Verification items for the finished model (mm, model axes). Round coordinates to 2 decimals unless told otherwise and drop trailing zeros. Order: outer loops, then holes, each group sorted by start corner. A loop starts at its lowest first (then second) coordinate and runs counter-clockwise, first axis right, second up. Notation, with made-up numbers: M -12,59 L 10,59 A27 ccw 10,96 Z; hole C 80,15 d2. An arc over 180 degrees is marked long. Use one line per item in the form item = value. Start each with the question number.
Item 1: Cross-section at A-A on z = -2. Enter the section's corners in (x, y).
Item 2: Thickness scan on probe 1 along Z at (x, y) = (249.5, -5); probe 2 along Y at (x, z) = (0, -29.35); probe 3 along Y at (x, z) = (-298.5, -6). Record the ranges inside material, lowest first. Write a range as [from, to].
Item 3: Cross-section at B-B on x = 680. Enter the section's corners in (y, z).
Item 4: Cross-section at C-C on x = -46. Enter the section's corners in (y, z).
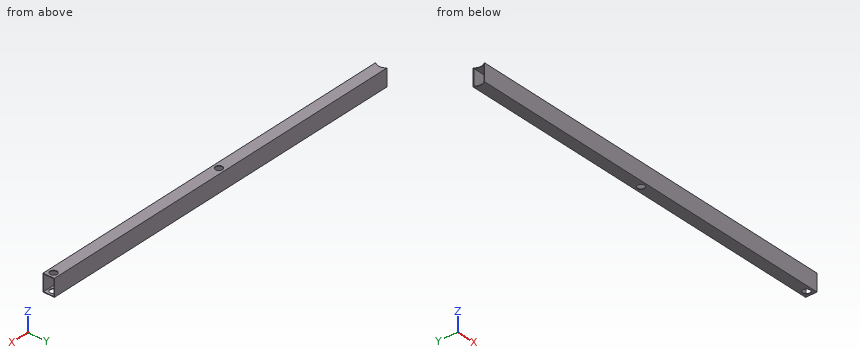
from build123d import *

# Parameters (mm, degrees)
SKETCH1_R           = 12.5
BOSS_EXTRUDE1_DEPTH = 30
SKETCH2_W           = 56
SKETCH2_H           = 36
CUT_EXTRUDE1_DEPTH  = 1368.639320225


with BuildPart() as part:
    # Sketch1 → Boss-Extrude1 (new body, symmetric)
    with BuildSketch(Plane.XY):
        with BuildLine():
            Line((700, -20), (700, 20))
            Line((700, 20), (-667.639320225, 20))
            ThreePointArc((-667.639320225, 20), (-661.974829231, 10.704662693), (-660, 0))
            ThreePointArc((-660, 0), (-661.974829231, -10.704662693), (-667.639320225, -20))
            Line((-667.639320225, -20), (700, -20))
        make_face()
        Circle(SKETCH1_R, mode=Mode.SUBTRACT)
        with Locations((680, 0)):
            Circle(SKETCH1_R, mode=Mode.SUBTRACT)
    extrude(amount=BOSS_EXTRUDE1_DEPTH, both=True)

    # Sketch2 → Cut-Extrude1 (cut, through all)
    with BuildSketch(Plane(origin=(700, 0, 0), x_dir=(0, 0, -1), z_dir=(1, 0, 0))):
        Rectangle(SKETCH2_W, SKETCH2_H)
    extrude(amount=-CUT_EXTRUDE1_DEPTH, mode=Mode.SUBTRACT)


solid = part.part
Output values:
q1.outline = M -667.64,-20 L 700,-20 L 700,-18 L -666,-18 A30 cw Z; M -667.64,20 A30 cw -666,18 L 700,18 L 700,20 Z
q2.probe_1 = [-30, -28], [28, 30]
q2.probe_2 = [-20, -12.5], [12.5, 20]
q2.probe_3 = [-20, -18], [18, 20]
q3.outline = M -20,-30 L -12.5,-30 L -12.5,-28 L -18,-28 L -18,28 L -12.5,28 L -12.5,30 L -20,30 Z; M 12.5,-30 L 20,-30 L 20,30 L 12.5,30 L 12.5,28 L 18,28 L 18,-28 L 12.5,-28 Z
q4.outline = M -20,-30 L 20,-30 L 20,30 L -20,30 Z; hole M -18,-28 L 18,-28 L 18,28 L -18,28 Z
